Here's how the part is built. I have some questions about the finished solid (model axes, mm). A direction names the side the tool comes from. Give positions to 0.01 mm unless a question says otherwise; leave off trailing zeros. Order: outer loops, then holes, each group sorted by start corner. A loop starts at its lowest first (then second) coordinate and runs counter-clockwise, first axis right, second up.
from build123d import *

# Parameters (mm, degrees)
F2_R = 0.8
F3_R = 3


with BuildPart() as f1:
    # F0 (on Front) → F1 (revolve)
    with BuildSketch(Plane.XZ):
        Polygon((66.5, 40.850982), (55.8942, 40.850982), (50.126342, -38.021039), (54, -38.021039), (54, -39.021039), (57, -39.021039), (57, -38.021039), (59.5, -38.021039), (59.5, -35.521039), (53.5, -33.021039), (58.5, 35.350982), (66.5, 38.850982), align=None)
    revolve(axis=Axis((0, 0, -10.226812), (0, 0, -1)))

    # F2
    f2_edges = [f1.edges().sort_by_distance(p)[0] for p in [
        (-54, 0, -39.021039),
        (-57, 0, -39.021039),
    ]]
    fillet(f2_edges, radius=F2_R)

    # F3
    f3_edges = [f1.edges().sort_by_distance(p)[0] for p in [
        (-58.5, 0, 35.350982),
        (-53.5, 0, -33.021039),
    ]]
    fillet(f3_edges, radius=F3_R)


solid = f1.part
Q1. If we section it at B-B on z = -6.5: List the corners of the cut face in (x, y) for me.
Filled sheet:
outline: circle Ø110.88 at (0, 0); hole circle Ø104.86 at (0, 0)
Q2. For faces 1 (the face through (-12, 54, -39.021)), 2 (the face through (31.99, -50.17, -36.75)), 3 (the face through (-7.23, -55.05, -5.36)), which set-ups out of +Z, -Z, +X, -X, +Y, -Y let a thin tool reach every point of the face, with its end or its side?
Filled sheet:
face 1: -Z, +X, -X, +Y, -Y
face 2: -Z
face 3: none
Q3. I need wall thicknesses on L1, parallel to X at y = 0, z = -38.1; L2, parallel to X at y = -17.5, z = 30.5; L3, parallel to Y at x = -41, z = 27. Which ranges of each line are inside material? Lowest first, please.
Filled sheet:
L1: x = -57 to -54, 54 to 57
L2: x = -55.45 to -52.29, 52.29 to 55.45
L3: y = -40.87 to -36.48, 36.48 to 40.87
Q4. If we section it at A-A on z = -15: List the corners of the cut face in (x, y) for me, plus the area to 3 significant figures.
Filled sheet:
outline: circle Ø109.64 at (0, 0); hole circle Ø103.62 at (0, 0)
area: 1,010 mm2
Q5. I'm going to push flat-ended pins straight in: P1, Ø12, axis at x = -44.5, z = 18.5, coming from the +Y side; P2, Ø10, axis at y = 12, z = 8, coming from the -X side; P3, Ø8, axis at x = 10.5, z = -9.5, coming from the -Y side. Where does each tip first touch, or does it pass through?
Filled sheet:
P1: stops at y = 42.43
P2: stops at x = -56.16
P3: stops at y = -54.92
Q6. Thinking about a two-plate mould opening in X: for faces 4 (the face through (-11.48, 51.71, 0.86)), 5 (the face through (25.698, 49.407, -33.934)), 6 (the face through (-15, -54, 40.851)), which applies, released by +X, released by -X, zero draft, split by the parting line, or undercut?
Filled sheet:
face 4: undercut
face 5: split by the parting line
face 6: zero draft
